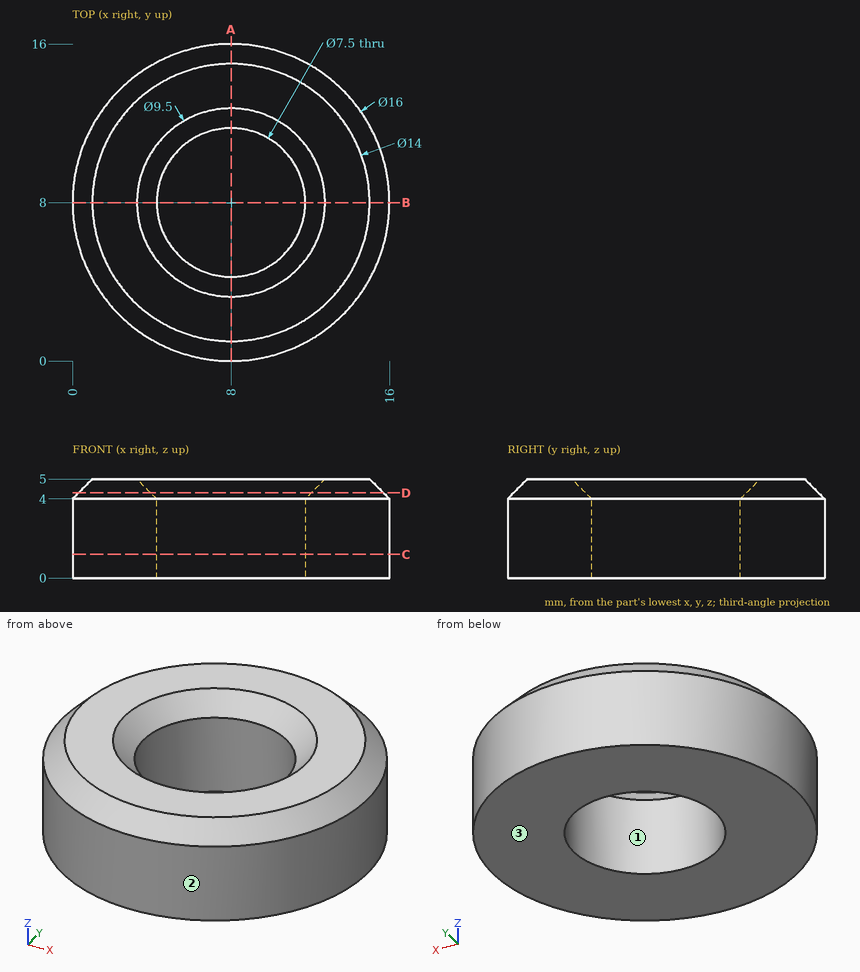
Could you check a few things on this drawing? It's one solid part, dimensions in mm from its lowest x, y, z. Coordinates: 2 decimals unless noted, no trailing zeros. Loops run counter-clockwise (first coordinate to the right, second up) from the corner with the lowest first, then second, coordinate; pieces in that order, holes last.
1. I need wall thicknesses on L1, parallel to Y at x = 8, z = 2.8; L2, parallel to Y at x = 10.5, z = 2.3; L3, parallel to X at y = 5.25, z = 2.7. Which ranges of each line are inside material? Lowest first, please.
2. We'd pull the mould along X, two halves only. Please class the marked faces 1, 2 and 3: released by +X, released by -X, zero draft, split by the parting line, or undercut.
3. For P1, Ø4.5, axis at x = 8, y = 8, coming from the +Z side; P2, Ø2, axis at x = 5.5, z = 1, coming from the +Y side; P3, Ø1, axis at y = 12, z = 3.5, coming from the -X side, each with a flat end and sliding along its axis, tell me the tip position at first contact or that it passes through.
4. Imagine slicing it at C-C (z = 1.2). Please give me the cut outline in (x, y), and give its area (3 significant figures).
5. Imagine slicing it at A-A (x = 8). Please give me the cut outline in (y, z).
6. Imagine slicing it at D-D (z = 4.3). Please give me the cut outline in (x, y), and give its area (3 significant figures).
Computed values:
1. L1: y = 0 to 4.25, 11.75 to 16
1. L2: y = 0.4 to 5.2, 10.8 to 15.6
1. L3: x = 0.49 to 5.45, 10.55 to 15.51
2. face 1: undercut
2. face 2: split by the parting line
2. face 3: zero draft
3. P1: passes through
3. P2: stops at y = 15.86
3. P3: stops at x = 0.81
4. outline: circle Ø16 at (8, 8); hole circle Ø7.5 at (8, 8)
4. area: 157 mm2
5. outline: (0, 0) - (4.25, 0) - (4.25, 4) - (3.25, 5) - (1, 5) - (0, 4) - close; (11.75, 0) - (16, 0) - (16, 4) - (15, 5) - (12.75, 5) - (11.75, 4) - close
6. outline: circle Ø15.4 at (8, 8); hole circle Ø8.1 at (8, 8)
6. area: 135 mm2
